Can you work these out from the model? Positions are in its coordinate system, mm. Face numbers are marked on the shaded views. A direction names the side the tool comes from. Give positions to 0.01 mm unless a question says otherwise; leave off trailing zeros. Write each loop counter-clockwise with the first axis right and the second up, starting at its lowest first coordinate (ties: lowest second). Pieces come first, ordered by that corner, then holes. Notation, with made-up numbers: M 52,24.25 L 62,24.25 A24 ccw 62,34.25 Z; hole C 11,63.25 d9. An arc over 180 degrees is marked long. Write each question's results on one line, items separated by ' | '.
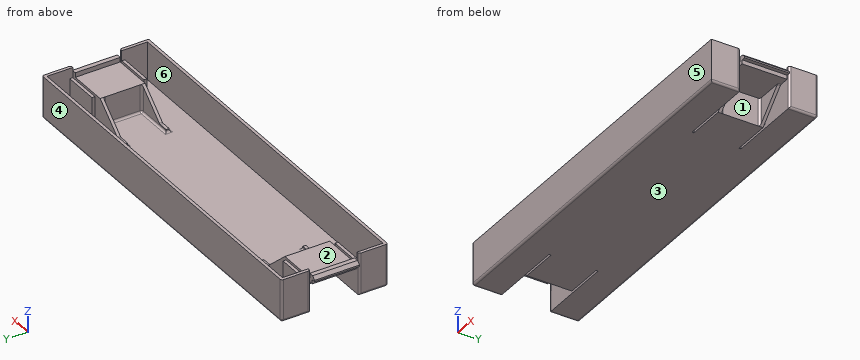
from build123d import *

# Parameters (mm, degrees)
PAD_DEPTH    = 1.6
SKETCH002_W  = 2
SKETCH002_H  = 17.7
PAD001_DEPTH = 11
PAD002_DEPTH = 4
SKETCH004_W  = 15
SKETCH004_H  = 17.7
PAD003_DEPTH = 1.6
SKETCH005_W  = 3
SKETCH005_H  = 17.7
PAD004_DEPTH = 1.8
PAD005_DEPTH = 1.2
PAD006_DEPTH = 1.2
CHAMFER_SIZE = 1.2
FILLET_R     = 0.8


with BuildPart() as part:
    # Sketch001 → Pad (new body)
    with BuildSketch(Plane.XY):
        Polygon((-44.5, -9.65), (-74.5, -9.65), (-74.5, -21), (74.5, -21), (74.5, -9.65), (44.5, -9.65), (44.5, -8.85), (59.5, -8.85), (59.5, 8.85), (44.5, 8.85), (44.5, 9.65), (74.5, 9.65), (74.5, 21), (-74.5, 21), (-74.5, 9.65), (-44.5, 9.65), (-44.5, 8.85), (-59.5, 8.85), (-59.5, -8.85), (-44.5, -8.85), align=None)
    extrude(amount=PAD_DEPTH)

    # Sketch002 → Pad001 (join)
    with BuildSketch(Plane.XY.offset(1.6)):
        Polygon((59.5, 9.65), (74.5, 9.65), (74.5, 21), (-74.5, 21), (-74.5, 9.65), (-59.5, 9.65), (-59.5, 10.85), (-73.3, 10.85), (-73.3, 19.8), (73.3, 19.8), (73.3, 10.85), (59.5, 10.85), align=None)
        Polygon((-59.5, -9.65), (-74.5, -9.65), (-74.5, -21), (74.5, -21), (74.5, -9.65), (59.5, -9.65), (59.5, -10.85), (73.3, -10.85), (73.3, -19.8), (-73.3, -19.8), (-73.3, -10.85), (-59.5, -10.85), align=None)
        with Locations((-58.5, 0)):
            Rectangle(SKETCH002_W, SKETCH002_H)
        with Locations((58.5, 0)):
            Rectangle(SKETCH002_W, SKETCH002_H)
    extrude(amount=PAD001_DEPTH)

    # Sketch003 → Pad002 (join)
    with BuildSketch(Plane.XY.offset(12.6)):
        Polygon((-74.5, 9.65), (-74.5, 21), (74.5, 21), (74.5, 9.65), (73.3, 9.65), (73.3, 19.8), (-73.3, 19.8), (-73.3, 9.65), align=None)
        Polygon((-74.5, -9.65), (-74.5, -21), (74.5, -21), (74.5, -9.65), (73.3, -9.65), (73.3, -19.8), (-73.3, -19.8), (-73.3, -9.65), align=None)
    extrude(amount=PAD002_DEPTH)

    # Sketch004 → Pad003 (join)
    with BuildSketch(Plane.XY.offset(12.6)):
        with Locations((-67, 0)):
            Rectangle(SKETCH004_W, SKETCH004_H)
        with Locations((67, 0)):
            Rectangle(SKETCH004_W, SKETCH004_H)
    extrude(amount=-PAD003_DEPTH)

    # Sketch005 → Pad004 (join)
    with BuildSketch(Plane.XY.offset(12.6)):
        with Locations((-74.5, 0)):
            Rectangle(SKETCH005_W, SKETCH005_H)
        with Locations((74.5, 0)):
            Rectangle(SKETCH005_W, SKETCH005_H)
    extrude(amount=PAD004_DEPTH)

    # Sketch006 (on DatumPlane) → Pad005 (join)
    with BuildSketch(Plane(origin=(59.5, 8.85, 0), x_dir=(-1, 0, 0), z_dir=(0, 1, 0))):
        Polygon((2, 1.6), (17, 1.6), (17, 2.8), (13, 2.8), (2, 12.6), align=None)
        Polygon((0, 0), (0, 11), (-11, 11), align=None)
        Polygon((119, 0), (119, 11), (130, 11), align=None)
        Polygon((102, 1.6), (117, 1.6), (117, 12.6), (106, 2.8), (102, 2.8), align=None)
    extrude(amount=-PAD005_DEPTH)

    # Sketch007 (on DatumPlane) → Pad006 (join)
    with BuildSketch(Plane(origin=(59.5, -8.85, 0), x_dir=(-1, 0, 0), z_dir=(0, 1, 0))):
        Polygon((2, 1.6), (17, 1.6), (17, 2.8), (13, 2.8), (2, 12.6), align=None)
        Polygon((0, 0), (0, 11), (-11, 11), align=None)
        Polygon((119, 0), (119, 11), (130, 11), align=None)
        Polygon((102, 1.6), (117, 1.6), (117, 12.6), (106, 2.8), (102, 2.8), align=None)
    extrude(amount=PAD006_DEPTH)

    # Chamfer
    chamfer_edges = [part.edges().sort_by_distance(p)[0] for p in [
        (76, 0, 14.4),
        (-76, 0, 14.4),
    ]]
    chamfer(chamfer_edges, length=CHAMFER_SIZE)

    # Fillet
    fillet_edges = [part.edges().sort_by_distance(p)[0] for p in [
        (43.5, 8.85, 1.6),
        (-43.5, 8.85, 1.6),
        (-42.5, 8.25, 1.6),
        (-42.5, -8.25, 1.6),
        (-50, -7.65, 1.6),
        (-57.5, 0, 1.6),
        (50, -7.65, 1.6),
        (42.5, 8.25, 1.6),
        (50, 7.65, 1.6),
        (57.5, 0, 1.6),
        (42.5, -8.25, 1.6),
        (43.5, -8.85, 1.6),
        (-43.5, -8.85, 1.6),
        (-50, 7.65, 1.6),
        (74.5, 21, 8.3),
        (-74.5, 21, 8.3),
        (-74.5, 15.325, 0),
        (-74.5, 9.65, 8.3),
        (-74.5, -9.65, 8.3),
        (-74.5, -15.325, 0),
        (-74.5, -21, 8.3),
        (0, 21, 0),
        (0, -21, 0),
        (-59.5, 7.65, 5.5),
        (-59.5, -7.65, 5.5),
        (74.5, 15.325, 0),
        (74.5, 9.65, 8.3),
        (74.5, -15.325, 0),
        (74.5, -9.65, 8.3),
        (59.5, 7.65, 5.5),
        (59.5, -7.65, 5.5),
        (70.5, -8.25, 11),
        (70.5, 8.25, 11),
        (-70.5, 8.25, 11),
        (-70.5, -8.25, 11),
        (-57.5, 7.65, 7.1),
        (57.5, 7.65, 7.1),
        (57.5, -7.65, 7.1),
        (-57.5, -7.65, 7.1),
        (-46.5, -8.25, 2.8),
        (-46.5, 8.25, 2.8),
        (46.5, 8.25, 2.8),
        (46.5, -8.25, 2.8),
    ]]
    fillet(fillet_edges, radius=FILLET_R)


solid = part.part
Item 1: I want a section at B-B, the plane y = -5. Please give me the cut outline in (x, z).
Geometry says:
outline: M -76,12.6 L -74.5,12.6 L -74.5,11 L -59.5,11 L -59.5,0 L 59.5,0 L 59.5,11 L 74.5,11 L 74.5,12.6 L 76,12.6 L 76,13.2 L 74.8,14.4 L 73,14.4 L 73,12.6 L 57.5,12.6 L 57.5,2.4 A0.8 cw 56.7,1.6 L -56.7,1.6 A0.8 cw -57.5,2.4 L -57.5,12.6 L -73,12.6 L -73,14.4 L -74.8,14.4 L -76,13.2 Z
Item 2: If I drill on line 1 (Y direction, x = 55, z = 6); line 2 (Y direction, x = 61, z = 15); line 3 (X direction, y = -3, z = 6.5), over which ranges is the centre line in solid material (lowest first)? Write a range as from..to.
Geometry says:
line 1: y = -21..-19.8, -8.85..-7.65, 7.65..8.85, 19.8..21 | line 2: y = -21..-19.8, 19.8..21 | line 3: x = -59.5..-57.5, 57.5..59.5
Item 3: For the marked faces 1 and 2, which set-ups out of +Z, -Z, +X, -X, +Y, -Y let a thin tool reach every point of the face, with its end or its side?
Geometry says:
face 1: -Z, +X | face 2: +Z
Item 4: I'm going to push flat-ended pins straight in: pin 1 (4 mm diameter, centred on y = 8, z = 13.5, fed in from -X); pin 2 (1.3 mm diameter, centred on y = 0.5, z = 11.5, fed in from -X); pin 3 (1 mm diameter, centred on x = 69.5, y = 10.5, fed in from +Z); pin 4 (0.6 mm diameter, centred on x = -45, y = 8.5, fed in from +Z). Where does each tip first touch, or does it pass through?
Geometry says:
pin 1: stops at x = -76 | pin 2: stops at x = -74.5 | pin 3: stops at z = 12.6 | pin 4: stops at z = 2.8
Item 5: I want a section at D-D, the plane z = 5.75. Give the number of separate pieces and of enclosed holes in the cut face, and give its area (3 significant figures).
Geometry says:
separate pieces: 4 | enclosed holes: 0 | area: 608 mm2
Item 6: I want a section at A-A, the plane x = -62. Please give me the cut outline in (y, z), and give its area (3 significant figures).
Geometry says:
outline: M -21,0.8 A0.8 ccw -20.2,0 L -9.65,0 L -9.65,12.6 L -10.85,12.6 L -10.85,1.6 L -19.8,1.6 L -19.8,16.6 L -21,16.6 Z; M -8.85,2.5 L -7.65,2.5 L -7.65,11 L 7.65,11 L 7.65,2.5 L 8.85,2.5 L 8.85,12.6 L -8.85,12.6 Z; M 9.65,0 L 20.2,0 A0.8 ccw 21,0.8 L 21,16.6 L 19.8,16.6 L 19.8,1.6 L 10.85,1.6 L 10.85,12.6 L 9.65,12.6 Z | area: 147 mm2
Item 7: Thinking about a two-plate mould opening in Y: for the marked faces 3, 4, 5 and 6, which applies, +Y half, -Y half, draft (parallel to the pull), parting line (faces both ways), or undercut?
Geometry says:
face 3: draft | face 4: +Y half | face 5: -Y half | face 6: undercut
Item 8: I want a section at C-C, the plane x = 34. Please give me the cut outline in (y, z).
Geometry says:
outline: M -21,0.8 A0.8 ccw -20.2,0 L 20.2,0 A0.8 ccw 21,0.8 L 21,16.6 L 19.8,16.6 L 19.8,1.6 L -19.8,1.6 L -19.8,16.6 L -21,16.6 Z
